from build123d import *

# Parameters (mm, degrees)
SKETCH1_W           = 41.303343927
SKETCH1_H           = 44.031810838
SKETCH1_R           = 11.8999
SKETCH1_R_2         = 2.54
BOSS_EXTRUDE1_DEPTH = 6.35


with BuildPart() as part:
    # Sketch1 → Boss-Extrude1 (new body)
    with BuildSketch(Plane.XY):
        with Locations((3.992518762, -3.025665718)):
            Rectangle(SKETCH1_W, SKETCH1_H)
        Circle(SKETCH1_R, mode=Mode.SUBTRACT)
        with Locations((19.05, 7.874)):
            Circle(SKETCH1_R_2, mode=Mode.SUBTRACT)
        with Locations((19.05, -19.05)):
            Circle(SKETCH1_R_2, mode=Mode.SUBTRACT)
        with Locations((-7.874, -19.05)):
            Circle(SKETCH1_R_2, mode=Mode.SUBTRACT)
    extrude(amount=BOSS_EXTRUDE1_DEPTH)


solid = part.part
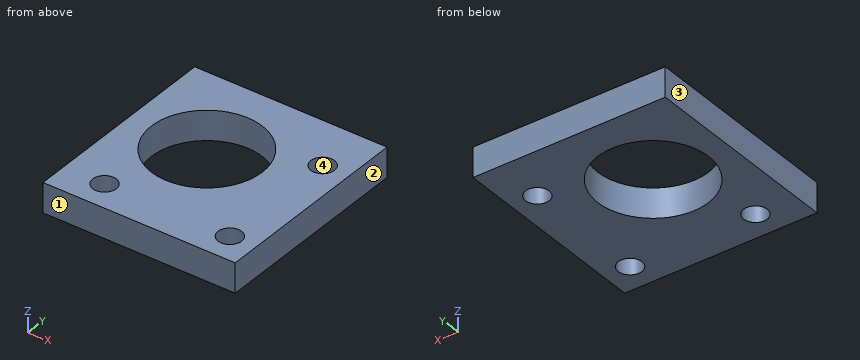
Input: part model. Units: mm. Frame: model coordinates. Face numbers are marked on the shaded views. Give positions to 0.01 mm unless a question says otherwise; leave off trailing zeros. Loops run counter-clockwise (first coordinate to the right, second up) from the corner with the lowest first, then second, coordinate; pieces in that order, holes last. Notation, with made-up numbers: M 81,-11.75 L 95,-11.75 A21 ccw 95,13.25 Z; hole C 84,72.5 d11. An arc over 180 degrees is marked long. Use CSV: the item, a comma, the result in double quotes.
(1) Pull-direction query (X, two-part tool) for the marked faces 1, 2, 3 and 4; classes: pulls with the +X half, pulls with the -X half, needs draft (parallel to the pull), parting line crosses it, or undercut.
Outcome:
face 1,"needs draft"
face 2,"pulls with the +X half"
face 3,"pulls with the -X half"
face 4,"undercut"
(2) Pin query (flat end, axial travel): P1, Ø8, axis at x = 19.05, y = 7.874, coming from the +Z side. Return the tip coordinate at first contact, or that it passes through.
Outcome:
P1,"stops at z = 6.35"
(3) Section D-D, the plane y = -19.05. Return loops of the section in (x, z), plus the area to 3 significant figures.
Outcome:
outline,"M -16.66,0 L -10.41,0 L -10.41,6.35 L -16.66,6.35 Z; M -5.33,0 L 16.51,0 L 16.51,6.35 L -5.33,6.35 Z; M 21.59,0 L 24.64,0 L 24.64,6.35 L 21.59,6.35 Z"
area,"198 mm²"
(4) Material intervals for L1, parallel to Y at x = 19.05, z = 1.75; L2, parallel to Y at x = 0, z = 2.25; L3, parallel to X at y = 0.5, z = 2.5, sorted ascending. Write a range as [from, to].
Outcome:
L1,"y = [-25.04, -21.59], [-16.51, 5.33], [10.41, 18.99]"
L2,"y = [-25.04, -11.9], [11.9, 18.99]"
L3,"x = [-16.66, -11.89], [11.89, 24.64]"
(5) Section A-A, the plane y = 0. Return loops of the section in (x, z), plus the area to 3 significant figures.
Outcome:
outline,"M -16.66,0 L -11.9,0 L -11.9,6.35 L -16.66,6.35 Z; M 11.9,0 L 24.64,0 L 24.64,6.35 L 11.9,6.35 Z"
area,"111 mm²"
(6) Section C-C, the plane x = 19.05. Return loops of the section in (y, z).
Outcome:
outline,"M -25.04,0 L -21.59,0 L -21.59,6.35 L -25.04,6.35 Z; M -16.51,0 L 5.33,0 L 5.33,6.35 L -16.51,6.35 Z; M 10.41,0 L 18.99,0 L 18.99,6.35 L 10.41,6.35 Z"
(7) Section B-B, the plane x = 0. Return loops of the section in (y, z), plus the area to 3 significant figures.
Outcome:
outline,"M -25.04,0 L -11.9,0 L -11.9,6.35 L -25.04,6.35 Z; M 11.9,0 L 18.99,0 L 18.99,6.35 L 11.9,6.35 Z"
area,"128 mm²"
